Answer from the drawing. Dimensions are ordinates in mm from the lowest x, y and z of the part. Give positions to 0.01 mm unless a question says otherwise; leave off trailing zeros. Loops run counter-clockwise (first coordinate to the right, second up) from the corner with the lowest first, then second, coordinate; pieces in that order, holes last. Notation, with made-up numbers: (10.5, 54) - (33.5, 54) arc R9 cw to (33.5, 63) - close; hole circle Ø6 at (40.25, -9.75). An arc over 180 degrees is marked (long way). Put each result on its own line as item: value. Start each with the question number.
1. Consider L1, parallel to X at y = 1.9, z = 42; L2, parallel to X at y = 0.25, z = 30; L3, parallel to Z at x = 13, y = 1.9. Determine where each line is inside the solid, lowest interval first. Write a range as from..to.
2. A cutting plane is placed at C-C, the plane x = 47.5. Determine the outline of the cut face in (y, z) (1 decimal).
3. A cutting plane is placed at D-D, the plane z = 16. Determine the outline of the cut face in (x, y) (1 decimal), plus the area to 3 significant figures.
4. A cutting plane is placed at A-A, the plane z = 39.5. Count the separate pieces of the cut face and the enclosed holes in it, plus the area to 3 significant figures.
5. Given pin 1 Ø1 at (y, z) = (1, 39.5) entering from -X; pin 2 Ø1.6 at (y, z) = (1.5, 35.5) entering from +X; pin 3 Ø1 at (x, y) = (41.5, 2) entering from +Z, each flat-ended and moving along its own axis, determine where each tip first touches the part or whether it passes through.
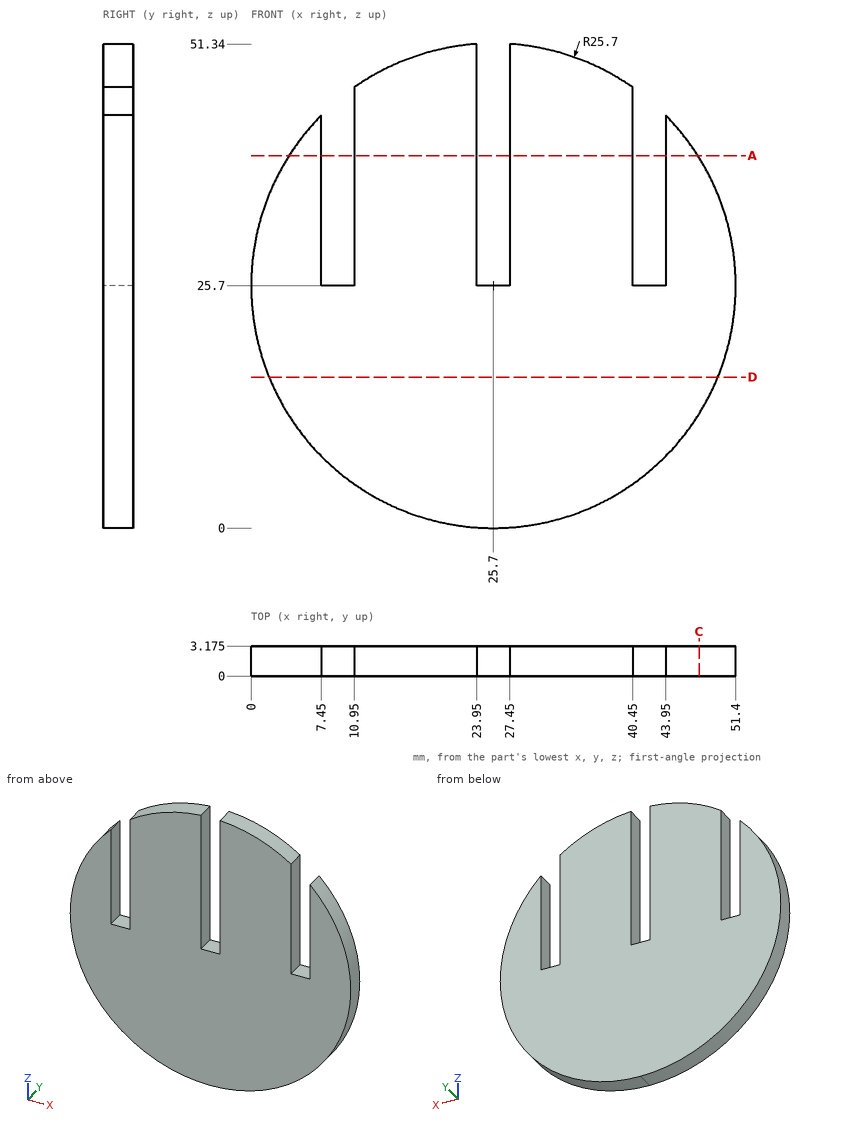
Return value:
1. L1: x = 5.83..7.45, 10.95..23.95, 27.45..40.45, 43.95..45.57
1. L2: x = 0.36..7.45, 10.95..23.95, 27.45..40.45, 43.95..51.04
1. L3: z = 3.36..48.04
2. outline: (0, 12.1) - (3.2, 12.1) - (3.2, 39.3) - (0, 39.3) - close
3. outline: (1.9, 0) - (49.5, 0) - (49.5, 3.2) - (1.9, 3.2) - close
3. area: 151 mm2
4. separate pieces: 4
4. enclosed holes: 0
4. area: 104 mm2
5. pin 1: stops at x = 3.71
5. pin 2: stops at x = 49.77
5. pin 3: stops at z = 25.7
